Could you check a few things on this model? Use its own coordinates, in mm. A direction names the side the tool comes from. Give positions to 0.01 mm unless a question says otherwise; leave off trailing zeros. Write each loop counter-clockwise with the first axis right and the second up, starting at its lowest first coordinate (ties: lowest second). Pieces come first, ordered by that corner, then holes. Notation, with made-up numbers: (72, 5) -> (99, 5) arc R35 ccw to (99, 37) -> close; hole circle Ø9 at (-28, 40.5). An arc over 180 degrees is marked (long way). Write item = value, one per line. Start each with the question number.
```python
from build123d import *

# Parameters (mm, degrees)
SKETCH_1_R      = 1.05
SKETCH_1_W      = 15
SKETCH_1_H      = 6
SKETCH_1_R_2    = 11
EXTRUDE_1_DEPTH = 1.6


with BuildPart() as part:
    # 草图1 → 凸台-拉伸1 (new body)
    with BuildSketch(Plane(origin=(0, 0, 0), x_dir=(1, 0, 0), z_dir=(0, 1, 0))):
        Polygon((47.5, 0), (0, 0), (0, -24), (10, -24), (10, -64), (14, -64), (14, -80.5), (19.5, -80.5), (19.5, -77.5), (25, -77.5), (25, -87.5), (20, -87.5), (20, -98.5), (0, -98.5), (0, -143), (99, -143), (99, -40), (88, -40), (88, -29.5), (99, -29.5), (99, -22), (88.5, -22), (88.5, 0), (80, 0), (80, -22), (71, -22), (71, 0), (62.5, 0), (62.5, -16.5), (47.5, -16.5), align=None)
        with Locations(Location((21.8, -94.8, 0), (0, 0, 270))):
            Circle(SKETCH_1_R, mode=Mode.SUBTRACT)
        with Locations((87.5, -90.5)):
            Rectangle(SKETCH_1_W, SKETCH_1_H, mode=Mode.SUBTRACT)
        with Locations(Location((94.8, -94.8, 0), (0, 0, 270))):
            Circle(SKETCH_1_R, mode=Mode.SUBTRACT)
        with Locations(Location((21.8, -26.8, 0), (0, 0, 270))):
            Circle(SKETCH_1_R, mode=Mode.SUBTRACT)
        with Locations(Location((7, -7, 0), (0, 0, 270))):
            Circle(SKETCH_1_R, mode=Mode.SUBTRACT)
        with Locations(Location((20, -12, 0), (0, 0, 270))):
            Circle(SKETCH_1_R, mode=Mode.SUBTRACT)
        Polygon((34.10303038, -60.69848481), (63.80151519, -31), (93.5, -60.69848481), (63.80151519, -90.39696962), align=None, mode=Mode.SUBTRACT)
        with Locations(Location((96.3, -55.2, 0), (0, 0, 270))):
            Circle(SKETCH_1_R, mode=Mode.SUBTRACT)
        with Locations(Location((94.8, -26.8, 0), (0, 0, 270))):
            Circle(SKETCH_1_R, mode=Mode.SUBTRACT)
        with Locations(Location((81.9, -4.6, 0), (0, 0, 270))):
            Circle(SKETCH_1_R, mode=Mode.SUBTRACT)
        with Locations(Location((87, -7, 0), (0, 0, 270))):
            Circle(SKETCH_1_R, mode=Mode.SUBTRACT)
        with Locations(Location((66, -106, 0), (0, 0, 270))):
            Circle(SKETCH_1_R, mode=Mode.SUBTRACT)
        with Locations(Location((7, -136, 0), (0, 0, 270))):
            Circle(SKETCH_1_R, mode=Mode.SUBTRACT)
        with Locations(Location((33, -132, 0), (0, 0, 270))):
            Circle(SKETCH_1_R, mode=Mode.SUBTRACT)
        with Locations(Location((33, -106, 0), (0, 0, 270))):
            Circle(SKETCH_1_R, mode=Mode.SUBTRACT)
        with Locations(Location((66, -132, 0), (0, 0, 270))):
            Circle(SKETCH_1_R, mode=Mode.SUBTRACT)
        with Locations(Location((49.5, -119, 0), (0, 0, 270))):
            Circle(SKETCH_1_R_2, mode=Mode.SUBTRACT)
        with Locations(Location((87, -136, 0), (0, 0, 270))):
            Circle(SKETCH_1_R, mode=Mode.SUBTRACT)
    extrude(amount=EXTRUDE_1_DEPTH)


solid = part.part
```
(1) I'm going to push flat-ended pins straight in: pin 1 (1.7 mm diameter, centred on x = 7, z = 7, fed in from +Y); pin 2 (0.8 mm diameter, centred on x = 94.5, y = 0.5, fed in from -Z); pin 3 (0.8 mm diameter, centred on y = 1, z = 72.5, fed in from -X). Where does each tip first touch, or does it pass through?
(2) We'd pull the mould along Z, two halves only. Please class faces 3 (the flat face through (49.16, 0.789, 75.756)), 4 (the flat face through (38, 0, 70)): released by +Z, released by -Z, zero draft, split by the parting line, or undercut.
(3) On a 3-axis mill with a long thin cutter (end or side, diameter ignored), from which of +Z, -Z, +X, -X, +Y, -Y can I reach the whole of each face in a straight line? I mean faces 1 (the flat face through (38, 1.6, 70)), 2 (the flat face through (78.4, 0.8, 45.6)). Say none if no direction works.
(4) Imagine slicing it at B-B (y = 0.7). State how many separate pieces and enclosed holes the cut face has, then the cut area to 3 significant figures.
(5) Imagine slicing it at A-A (x = 52). Please give me the cut outline in (y, z).
(6) If I drill on line 1 along X through (y, z) = (0.55, 132); line 2 along X through (y, z) = (1.25, 136); line 3 along X through (y, z) = (0.95, 4.6), over which ranges is the centre line in solid material (lowest first)? Write a range as from..to.
Answers below:
q1.pin_1 = through
q1.pin_2 = 22
q1.pin_3 = 14
q2.face_3 = undercut
q2.face_4 = zero draft
q3.face_1 = +Z, -Z, +X, -X, +Y
q3.face_2 = +Y, -Y
q4.separate_pieces = 1
q4.enclosed_holes = 18
q4.area = 10,000 mm^2
q5.outline = (0, 16.5) -> (1.6, 16.5) -> (1.6, 42.8) -> (0, 42.8) -> close; (0, 78.6) -> (1.6, 78.6) -> (1.6, 108.29) -> (0, 108.29) -> close; (0, 129.71) -> (1.6, 129.71) -> (1.6, 143) -> (0, 143) -> close
q6.line_1 = 0..31.95, 34.05..64.95, 67.05..99
q6.line_2 = 0..5.95, 8.05..85.95, 88.05..99
q6.line_3 = 0..47.5, 62.5..71, 80..80.85, 82.95..88.5
